Input: part model. Units: mm. Frame: model coordinates. Round coordinates to 2 decimals unless told otherwise and drop trailing zeros. Loops run counter-clockwise (first coordinate to the right, second up) from the corner with the lowest first, then second, coordinate; pieces in that order, holes last. Notation, with made-up numbers: (20.5, -1.75) - (55.5, -1.75) arc R25 ccw to (55.5, 37.25) - close; hole circle Ø3 at (6.25, 59.25). An arc over 180 degrees is marked (long way). Use CSV: the item, a comma, the result in double quotes. Start each with the question number.
1. Material intervals for probe 1 along Z at (x, y) = (232.5, 15.25); probe 2 along Y at (x, z) = (63, -27.5); probe 3 along Y at (x, z) = (282, -36), sorted ascending. Write a range as from..to.
2. Cut plane A-A (x = 257). Return loops of the section in (y, z).
3. Pin query (flat end, axial travel): P1, Ø2, axis at x = 460, y = 14, coming from the -Z side; P2, Ø1, axis at x = 199, y = 3, coming from the -Z side; P3, Ø4, axis at x = 362.5, z = -67.5, coming from the -Y side. Return the tip coordinate at first contact, or that it passes through.
4. Cut plane B-B (z = -76.5). Return loops of the section in (x, y).
5. Cut plane C-C (y = 7). Return loops of the section in (x, z), and give its area (3 significant figures).
```python
from build123d import *

# Parameters (mm, degrees)
SKETCH1_W           = 514.35
SKETCH1_H           = 203.2
BOSS_EXTRUDE1_DEPTH = 19.05
CUT_EXTRUDE3_DEPTH  = 781.686405159


with BuildPart() as part:
    # Sketch1 → Boss-Extrude1 (new body)
    with BuildSketch(Plane(origin=(0, 0, 0), x_dir=(1, 0, 0), z_dir=(0, 1, 0))):
        with Locations((257.175, 101.6)):
            Rectangle(SKETCH1_W, SKETCH1_H)
    extrude(amount=BOSS_EXTRUDE1_DEPTH)

    # Sketch5 → Cut-Extrude3 (cut)
    with BuildSketch(Plane(origin=(514.35, 0, 0), x_dir=(0, 0, -1), z_dir=(1, 0, 0))):
        Polygon((0, 19.05), (4.561624762, 19.05), (3.848243249, 13.769669769), (105.769027955, 0), (0, 0), align=None)
        Polygon((203.2, 19.05), (200.626312897, 0), (203.2, 0), align=None)
    extrude(amount=-CUT_EXTRUDE3_DEPTH, mode=Mode.SUBTRACT)


solid = part.part
```
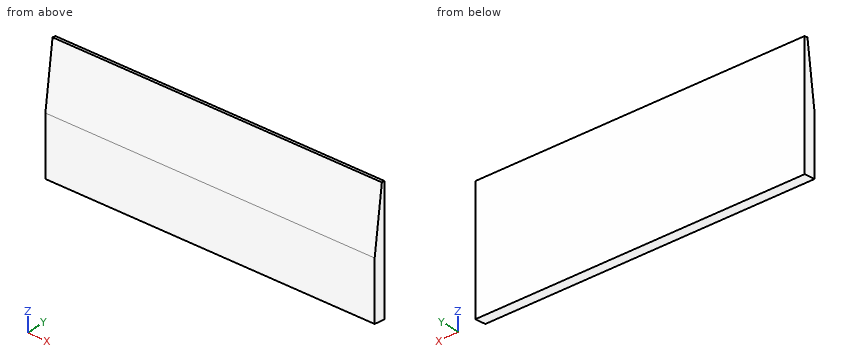
Established:
1,probe 1,"z = -202.69..-4.05"
1,probe 2,"y = 10.57..19.05"
1,probe 3,"y = 9.43..19.05"
2,outline,"(0, -200.63) - (19.05, -203.2) - (19.05, -4.56) - (13.77, -3.85) - (0, -105.77) - close"
3,P1,"stops at z = -202.65"
3,P2,"stops at z = -201.1"
3,P3,"stops at y = 4.9"
4,outline,"(0, 3.95) - (514.35, 3.95) - (514.35, 19.05) - (0, 19.05) - close"
5,outline,"(0, -201.57) - (514.35, -201.57) - (514.35, -53.96) - (0, -53.96) - close"
5,area,"75,900 mm2"
